Geometry check sheet. Reference: the model listing, model coordinates, mm. Face numbers are marked on the shaded views. Round coordinates to 2 decimals unless told otherwise and drop trailing zeros. Order: outer loops, then holes, each group sorted by start corner. A loop starts at its lowest first (then second) coordinate and runs counter-clockwise, first axis right, second up.
(1) Sectioned sample at A-A (z = 26.5). Record the boundary of the cut face in (x, y).
(2) Sectioned sample at B-B (x = -33). Record the boundary of the cut face in (y, z), plus the area to 3 significant figures.
(3) Release check for a two-part mould opening along X. For the marked faces 1 and 2 record: +X half, -X half, draft (parallel to the pull), parting line (faces both ways), or undercut.
(4) Material ranges on line 1 along X through (y, z) = (2.5, 42); line 2 along Z through (x, y) = (-28, 2.25); line 3 along Y through (x, z) = (-3, 29.5), recorded low to high.
(5) Go/stop test with flat-tipped pins: pin 1 (2 mm diameter, centred on x = -32.5, z = -13.5, fed in from -Y); pin 2 (8 mm diameter, centred on x = -10.5, y = 9.5, fed in from +Z); pin 3 (4.5 mm diameter, centred on y = 4.5, z = 10, fed in from +X); pin 4 (3 mm diameter, centred on x = 0.5, y = 4, fed in from -Z). Record where each tip stops, or that it passes through.
Autodesk Inventor part; units mm, degrees
ref_plane "YZ Plane" through (0, 0, 0) normal (1, 0, 0) x (0, 1, 0)
ref_plane "XZ Plane" through (0, 0, 0) normal (0, 1, 0) x (-1, 0, 0)
ref_plane "XY Plane" through (0, 0, 0) normal (0, 0, 1) x (1, 0, 0)
sketch "Master_XZ" plane through (0, 0, 0) normal (0, 1, 0) x (-1, 0, 0)
  line L0 (52.5, 47.5) -> (-52.5, 47.5)
  line L1 (-52.5, 47.5) -> (-52.5, -47.5)
  line L2 (-52.5, -47.5) -> (52.5, -47.5)
  line L3 (52.5, -47.5) -> (52.5, 47.5)
  line L4 (52.5, 47.5) -> (-52.5, -47.5) construction
  line L5 (-52.5, 47.5) -> (52.5, -47.5) construction
  line L6 (50.5, 45.5) -> (-50.5, 45.5)
  line L7 (-50.5, 45.5) -> (-50.5, -45.5)
  line L8 (-50.5, -45.5) -> (50.5, -45.5)
  line L9 (50.5, -45.5) -> (50.5, 45.5)
  line L10 (48.5, 43.5) -> (-48.5, 43.5)
  line L11 (-48.5, 43.5) -> (-48.5, -43.5)
  line L12 (-48.5, -43.5) -> (48.5, -43.5)
  line L13 (48.5, -43.5) -> (48.5, 43.5)
  point P0 (0, 0)
  dimension "d0" = 2
  dimension "d1" = 2
  dimension "d10" = 105
  dimension "d15" = 95
extrude "Floor" add sketch "Master_XZ" along normal blind 2 contours L3 L2 L1 L0 | L9 L8 L7 L6 | L13 L12 L11 L10
extrude "Walls" add sketch "Master_XZ" along normal blind 6 contours L9 L8 L7 L6
sketch "Lip_profile" plane through (0, 1, -41.5) normal (1, 0, 0) x (0, 0, -1)
  line L0 (-87, 1) -> (-87, 5)
  circle A0 centre (-87, 4) radius 1
  line L1 (-87, 5) -> (4, 5)
  line L2 (-87, 5) -> (-87, 3)
  point P0 (-41.5, -1)
  dimension "d6" = 2
  dimension "d7" = 1
extrude "Lip" add sketch "Lip_profile" along normal mid plane 100
sketch "Sketch3" plane through (50, 1, -41.5) normal (1, 0, 0) x (0, 0, -1)
  line L0 (-87, 5) -> (-87, 3)
  line L1 (-87, 5) -> (-87, 3)
  arc A0 (-87, 5) -> (-87, 3) centre (-87, 4) ccw
  point P0 (-41.5, -1)
revolve "Lip_edge_right" add sketch "Sketch3" angle 90 about axis through (50, 6, 45.5) along (0, 1, 0)
sketch "Sketch4" plane through (-50, 1, -41.5) normal (-1, 0, 0) x (0, 0, 1)
  line L0 (87, 3) -> (87, 5)
  arc A0 (87, 3) -> (87, 5) centre (87, 4) ccw
  point P0 (41.5, -1)
revolve "Lip_edge_left" add sketch "Sketch4" angle 90 about axis through (-50, 4, 45.5) along (0, -1, 0)
pattern_circular "Circular Pattern1" count 2 over 360 about axis through (0, -10, 0) along (0, 1, 0) of "Lip", "Lip_edge_right", "Lip_edge_left"
sketch "Sketch6" plane through (0, 2, 0) normal (0, 1, 0) x (1, 0, 0)
  circle A0 centre (-44.4993, 6.9242) radius 0.6
  circle A1 centre (-29.2593, 6.9242) radius 0.6
  circle A2 centre (-29.2593, -38.7958) radius 0.6
  circle A3 centre (-44.4993, -38.7958) radius 0.6
  circle A4 centre (-29.2593, 6.9242) radius 1
  circle A5 centre (-44.4993, 6.9242) radius 1
  circle A6 centre (-44.4993, -38.7958) radius 1
  circle A7 centre (-29.2593, -38.7958) radius 1
  point P0 (0, 0)
  dimension "d18" = 1.2
  dimension "d19" = 1.2
  dimension "d20" = 1.2
  dimension "d21" = 1.2
  dimension "d22" = 45.72
  dimension "d23" = 15.24
  dimension "d26" = 0.4
  dimension "d27" = 0.4
  dimension "d28" = 0.4
  dimension "d29" = 0.4
extrude "Standoff_base" add sketch "Sketch6" along normal blind 10 contours A0 | A1 | A2 | A3 | A4 | A5 | A6 | A7
sketch "Sketch8" plane through (-44.4993, 12, -6.9242) normal (0, 1, 0) x (1, 0, 0)
  circle A0 centre (0, 0) radius 1
  circle A1 centre (15.24, 0) radius 1
  circle A2 centre (0, -45.72) radius 1
  circle A3 centre (15.24, -45.72) radius 1
  circle A4 centre (0, 0) radius 0.6
  circle A5 centre (15.24, 0) radius 0.6
  circle A6 centre (0, -45.72) radius 0.6
  circle A7 centre (15.24, -45.72) radius 0.6
  point P0 (44.4993, -6.9242)
  dimension "d32" = 0.4
  dimension "d33" = 0.4
  dimension "d34" = 0.4
  dimension "d35" = 0.4
extrude "Standoff_tip" add sketch "Sketch8" along normal blind 3 draft -5 contours A4 | A5 | A6 | A7
equation "\"d27\" = d26"
equation "\"d28\" = d26"
equation "\"d29\" = d26"
equation "\"d32\" = d26"
equation "\"d33\" = d26"
equation "\"d34\" = d26"
equation "\"d35\" = d26"
properties part number "BARB_bottom" material "ABS Plastic"
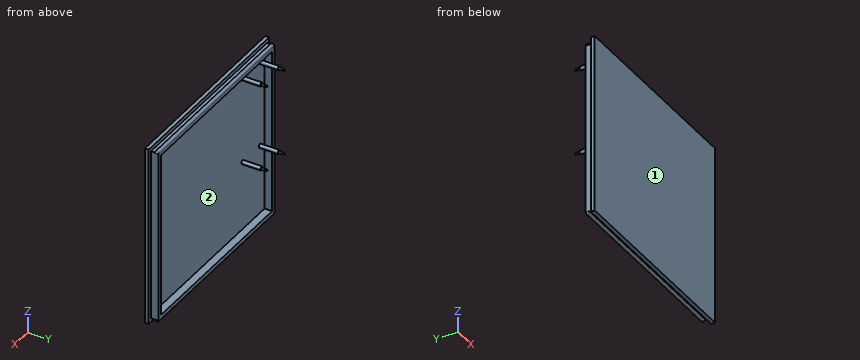
Answer below:
1. outline: (-52.5, 0) - (52.5, 0) - (52.5, 2) - (50.5, 2) - (50.5, 6) - (48.5, 6) - (48.5, 2) - (-48.5, 2) - (-48.5, 6) - (-50.5, 6) - (-50.5, 2) - (-52.5, 2) - close
2. outline: (0, -47.5) - (2, -47.5) - (2, -45.5) - (4, -45.5) arc R1 ccw to (6, -45.5) - (6, -43.5) - (2, -43.5) - (2, 43.5) - (6, 43.5) - (6, 45.5) arc R1 ccw to (4, 45.5) - (2, 45.5) - (2, 47.5) - (0, 47.5) - close
2. area: 209 mm2
3. face 1: draft
3. face 2: undercut
4. line 1: x = -50.5 to -48.5, 48.5 to 50.5
4. line 2: z = -45.5 to -43.5, 43.5 to 45.5
4. line 3: y = 0 to 2
5. pin 1: stops at y = 0
5. pin 2: stops at z = 46.37
5. pin 3: stops at x = 50.5
5. pin 4: stops at z = -46.5
